Source: CAD feature listing. Evaluate the final solid. Frame: model axes, mm. Face numbers are marked on the shaded views. A direction names the side the tool comes from. Round coordinates to 2 decimals unless told otherwise and drop trailing zeros. Write each loop counter-clockwise with the first axis right and the second up, starting at its lowest first coordinate (ties: lowest second). Pieces come first, ordered by that corner, then holes. Notation, with made-up numbers: M -38,26 L -5,26 A20 ccw -5,30 Z; hole C 71.5,87.25 d9. An arc over 180 degrees is marked long. Put each result on its own line as item: value. Start each with the question number.
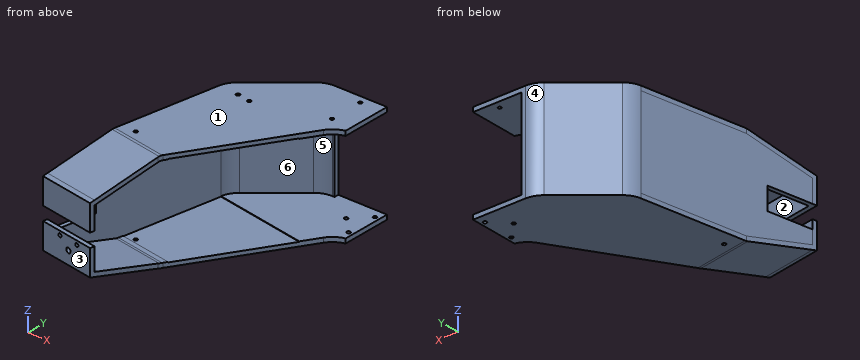
```python
from build123d import *

# Parameters (mm, degrees)
EXTRUDE_1_DEPTH      = 20
CUT_EXTRUDE_1_DEPTH  = 2
EXTRUDE_START        = 2
EXTRUDE_2_DEPTH      = 2
EXTRUDE_3_DEPTH      = 33
CUT_EXTRUDE_10_DEPTH = 22.5
EXTRUDE_4_DEPTH      = 25
SKETCH_19_W          = 6
SKETCH_19_H          = 22
CUT_EXTRUDE_11_DEPTH = 84.590810023
CUT_EXTRUDE_7_REACH  = 84.162
SKETCH_15_R          = 0.75
CUT_EXTRUDE_8_REACH  = 84.162
SKETCH_16_R          = 0.8
CUT_EXTRUDE_9_REACH  = 117.914
SKETCH_17_W          = 21.713584054
SKETCH_17_H          = 40
CUT_EXTRUDE_13_REACH = 84.162
SKETCH_23_R          = 0.8
SKETCH_24_R          = 0.8
CUT_EXTRUDE_14_DEPTH = 83.162435205
SKETCH_25_W          = 4
SKETCH_25_H          = 20
CUT_EXTRUDE_15_DEPTH = 82.996087258
CUT_EXTRUDE_16_REACH = 121.797
SKETCH_26_R          = 0.8
CUT_EXTRUDE_17_REACH = 121.797
SKETCH_27_R          = 1.1
FILLET_1_R           = 5
FILLET_2_R           = 5
FILLET_3_R           = 5
CUT_EXTRUDE_18_DEPTH = 20.2


with BuildPart() as part:
    # 草图1 → 凸台-拉伸1 (new, symmetric)
    with BuildSketch(Plane.XY):
        with BuildLine():
            Line((20.657346874, 53.638724152), (44.017644532, 53.638724152))
            Line((44.017644532, 53.638724152), (44.017644532, 51.638724152))
            Line((44.017644532, 51.638724152), (21.385287343, 51.638724152))
            ThreePointArc((21.385287343, 51.638724152), (17.96508591, 51.03565036), (14.957411246, 49.299168583))
            Line((14.957411246, 49.299168583), (-4.39648281, 33.059323219))
            ThreePointArc((-4.39648281, 33.059323219), (-6.628860751, 30.398878788), (-7.816684243, 27.135360565))
            Line((-7.816684243, 27.135360565), (-20.950105242, -47.347971173))
            Line((-20.950105242, -47.347971173), (-22.919720748, -47.000674818))
            Line((-22.919720748, -47.000674818), (-9.659894213, 28.199538337))
            ThreePointArc((-9.659894213, 28.199538337), (-8.472070721, 31.463056561), (-6.23969278, 34.123500992))
            Line((-6.23969278, 34.123500992), (14.229470778, 51.299168583))
            ThreePointArc((14.229470778, 51.299168583), (17.237145441, 53.03565036), (20.657346874, 53.638724152))
        make_face()
    extrude(amount=EXTRUDE_1_DEPTH, both=True)

    # 草图3 → 切除-拉伸1 (cut)
    with BuildSketch(Plane(origin=(-14.191017833, 2.502259328, 0), x_dir=(0, 0, 1), z_dir=(-0.9848077530122074, 0.17364817766693458, 0))):
        Polygon((13, -50.266596698), (20, -50.266596698), (20, -20.906299041), align=None)
    cut_extrude_1 = extrude(amount=-CUT_EXTRUDE_1_DEPTH, mode=Mode.SUBTRACT)

    # 镜向1: 切除-拉伸1 across plane
    add(cut_extrude_1.mirror(Plane.XY), mode=Mode.SUBTRACT)

    # 草图4 → 凸台-拉伸2 (add)
    with BuildSketch(Plane.XY.offset(20).offset(EXTRUDE_START)):
        with BuildLine():
            Line((44.017644532, 53.638724152), (44.017644532, 31.638724152))
            ThreePointArc((44.017644532, 31.638724152), (40.473292143, 30.034681338), (37.809285693, 27.199464091))
            Line((37.809285693, 27.199464091), (6.798835262, -22.427630496))
            Line((6.798835262, -22.427630496), (-17.821358564, -18.086426054))
            Line((-17.821358564, -18.086426054), (-9.659894213, 28.199538337))
            ThreePointArc((-9.659894213, 28.199538337), (-8.472070721, 31.463056561), (-6.23969278, 34.123500992))
            Line((-6.23969278, 34.123500992), (14.229470778, 51.299168583))
            ThreePointArc((14.229470778, 51.299168583), (17.237145441, 53.03565036), (20.657346874, 53.638724152))
            Line((20.657346874, 53.638724152), (44.017644532, 53.638724152))
        make_face()
    extrude_2 = extrude(amount=-EXTRUDE_2_DEPTH)

    # 草图5 → 凸台-拉伸3 (add)
    with BuildSketch(Plane(origin=(-14.191017833, 2.502259328, 0), x_dir=(0, 0, 1), z_dir=(-0.9848077530122074, 0.17364817766693458, 0))):
        Polygon((22, -20.906299041), (15, -50.266596698), (13, -50.266596698), (20, -20.906299041), align=None)
    extrude_3 = extrude(amount=-EXTRUDE_3_DEPTH)

    # 镜向3: 凸台-拉伸2, 凸台-拉伸3 across plane
    add(extrude_2.mirror(Plane.XY))
    add(extrude_3.mirror(Plane.XY))

    # 草图18 → 切除-拉伸10 (cut, symmetric)
    with BuildSketch(Plane.XY):
        Polygon((6.798835262, -22.427630496), (1.700473078, -51.34187926), (9.578935102, -52.731064681), (14.677297286, -23.816815917), align=None)
    extrude(amount=CUT_EXTRUDE_10_DEPTH, both=True, mode=Mode.SUBTRACT)

    # 草图10 → 凸台-拉伸4 (add)
    with BuildSketch(Plane(origin=(-14.191017833, 2.502259328, 0), x_dir=(0, 0, 1), z_dir=(-0.9848077530122074, 0.17364817766693458, 0))):
        Polygon((-15, -50.266596698), (15, -50.266596698), (14.523165597, -52.266596698), (-14.523165597, -52.266596698), align=None)
    extrude(amount=-EXTRUDE_4_DEPTH)

    # 草图19 → 切除-拉伸11 (cut, through all)
    with BuildSketch(Plane(origin=(-14.191017833, 2.502259328, 0), x_dir=(0, 0, 1), z_dir=(-0.9848077530122074, 0.17364817766693458, 0))):
        with Locations((0, -41.266596698)):
            Rectangle(SKETCH_19_W, SKETCH_19_H)
    extrude(amount=-CUT_EXTRUDE_11_DEPTH, mode=Mode.SUBTRACT)

    # 草图15 → 切除-拉伸7 (cut, up to next)
    with BuildSketch(Plane.XY.offset(22), mode=Mode.PRIVATE) as cut_extrude_7_sk1:
        with Locations((35.017644532, 50.138724152)):
            Circle(SKETCH_15_R)
    cut_extrude_7_tool1 = extrude(cut_extrude_7_sk1.sketch, amount=-CUT_EXTRUDE_7_REACH, mode=Mode.PRIVATE) & part.part
    # 草图15 → 切除-拉伸7 (cut, up to next)
    with BuildSketch(Plane.XY.offset(22), mode=Mode.PRIVATE) as cut_extrude_7_sk2:
        with Locations((35.017644532, 35.138724152)):
            Circle(SKETCH_15_R)
    cut_extrude_7_tool2 = extrude(cut_extrude_7_sk2.sketch, amount=-CUT_EXTRUDE_7_REACH, mode=Mode.PRIVATE) & part.part
    add(cut_extrude_7_tool1.solids().sort_by_distance((35.017645, 50.138724, 22))[0], mode=Mode.SUBTRACT)
    add(cut_extrude_7_tool2.solids().sort_by_distance((35.017645, 35.138724, 22))[0], mode=Mode.SUBTRACT)

    # 草图16 → 切除-拉伸8 (cut, up to next)
    with BuildSketch(Plane(origin=(0, 0, -22), x_dir=(-1, 0, 0), z_dir=(0, 0, -1)), mode=Mode.PRIVATE) as cut_extrude_8_sk1:
        with Locations((-42.017644532, 49.638724152)):
            Circle(SKETCH_16_R)
    cut_extrude_8_tool1 = extrude(cut_extrude_8_sk1.sketch, amount=-CUT_EXTRUDE_8_REACH, mode=Mode.PRIVATE) & part.part
    # 草图16 → 切除-拉伸8 (cut, up to next)
    with BuildSketch(Plane(origin=(0, 0, -22), x_dir=(-1, 0, 0), z_dir=(0, 0, -1)), mode=Mode.PRIVATE) as cut_extrude_8_sk2:
        with Locations((-42.017644532, 35.638724152)):
            Circle(SKETCH_16_R)
    cut_extrude_8_tool2 = extrude(cut_extrude_8_sk2.sketch, amount=-CUT_EXTRUDE_8_REACH, mode=Mode.PRIVATE) & part.part
    # 草图16 → 切除-拉伸8 (cut, up to next)
    with BuildSketch(Plane(origin=(0, 0, -22), x_dir=(-1, 0, 0), z_dir=(0, 0, -1)), mode=Mode.PRIVATE) as cut_extrude_8_sk3:
        with Locations((-35.017644532, 42.638724152)):
            Circle(SKETCH_16_R)
    cut_extrude_8_tool3 = extrude(cut_extrude_8_sk3.sketch, amount=-CUT_EXTRUDE_8_REACH, mode=Mode.PRIVATE) & part.part
    add(cut_extrude_8_tool1.solids().sort_by_distance((42.017645, 49.638724, -22))[0], mode=Mode.SUBTRACT)
    add(cut_extrude_8_tool2.solids().sort_by_distance((42.017645, 35.638724, -22))[0], mode=Mode.SUBTRACT)
    add(cut_extrude_8_tool3.solids().sort_by_distance((35.017645, 42.638724, -22))[0], mode=Mode.SUBTRACT)

    # 草图17 → 切除-拉伸9 (cut, up to next)
    with BuildSketch(Plane.XZ.offset(-51.638724152), mode=Mode.PRIVATE) as cut_extrude_9_sk1:
        with Locations((33.160852505, 0)):
            Rectangle(SKETCH_17_W, SKETCH_17_H)
    cut_extrude_9_tool1 = extrude(cut_extrude_9_sk1.sketch, amount=-CUT_EXTRUDE_9_REACH, mode=Mode.PRIVATE) & part.part
    add(cut_extrude_9_tool1.solids().sort_by_distance((33.160853, 51.638724, 0))[0], mode=Mode.SUBTRACT)

    # 草图23 → 切除-拉伸13 (cut, up to next)
    with BuildSketch(Plane.XY.offset(22), mode=Mode.PRIVATE) as cut_extrude_13_sk1:
        with Locations((-0.619145661, 27.643236889)):
            Circle(SKETCH_23_R)
    cut_extrude_13_tool1 = extrude(cut_extrude_13_sk1.sketch, amount=-CUT_EXTRUDE_13_REACH, mode=Mode.PRIVATE) & part.part
    # 草图23 → 切除-拉伸13 (cut, up to next)
    with BuildSketch(Plane.XY.offset(22), mode=Mode.PRIVATE) as cut_extrude_13_sk2:
        with Locations((5.289700857, 26.601347823)):
            Circle(SKETCH_23_R)
    cut_extrude_13_tool2 = extrude(cut_extrude_13_sk2.sketch, amount=-CUT_EXTRUDE_13_REACH, mode=Mode.PRIVATE) & part.part
    add(cut_extrude_13_tool1.solids().sort_by_distance((-0.619146, 27.643237, 22))[0], mode=Mode.SUBTRACT)
    add(cut_extrude_13_tool2.solids().sort_by_distance((5.289701, 26.601348, 22))[0], mode=Mode.SUBTRACT)

    # 草图24 → 切除-拉伸14 (cut, through all)
    with BuildSketch(Plane.XY.offset(22)):
        with Locations((-10.595826096, -14.770754093)):
            Circle(SKETCH_24_R)
    extrude(amount=-CUT_EXTRUDE_14_DEPTH, mode=Mode.SUBTRACT)

    # 草图25 → 切除-拉伸15 (cut, through all)
    with BuildSketch(Plane(origin=(-12.221402327, 2.154962972, 0), x_dir=(0, 0, -1), z_dir=(0.9848077530122075, -0.1736481776669347, 0))):
        with Locations((5, -40.266596698)):
            Rectangle(SKETCH_25_W, SKETCH_25_H)
    extrude(amount=-CUT_EXTRUDE_15_DEPTH, mode=Mode.SUBTRACT)

    # 草图26 → 切除-拉伸16 (cut, up to next)
    with BuildSketch(Plane(origin=(-9.075999269, -51.472549652, 0), x_dir=(0.9848077530122074, -0.17364817766693458, 0), z_dir=(-0.17364817766693458, -0.9848077530122074, 0)), mode=Mode.PRIVATE) as cut_extrude_16_sk1:
        with Locations((3.590062842, -4.75)):
            Circle(SKETCH_26_R)
    cut_extrude_16_tool1 = extrude(cut_extrude_16_sk1.sketch, amount=-CUT_EXTRUDE_16_REACH, mode=Mode.PRIVATE) & part.part
    # 草图26 → 切除-拉伸16 (cut, up to next)
    with BuildSketch(Plane(origin=(-9.075999269, -51.472549652, 0), x_dir=(0.9848077530122074, -0.17364817766693458, 0), z_dir=(-0.17364817766693458, -0.9848077530122074, 0)), mode=Mode.PRIVATE) as cut_extrude_16_sk2:
        with Locations((-5.409937158, -4.75)):
            Circle(SKETCH_26_R)
    cut_extrude_16_tool2 = extrude(cut_extrude_16_sk2.sketch, amount=-CUT_EXTRUDE_16_REACH, mode=Mode.PRIVATE) & part.part
    add(cut_extrude_16_tool1.solids().sort_by_distance((-5.540478, -52.095958, -4.75))[0], mode=Mode.SUBTRACT)
    add(cut_extrude_16_tool2.solids().sort_by_distance((-14.403747, -50.533124, -4.75))[0], mode=Mode.SUBTRACT)

    # 草图27 → 切除-拉伸17 (cut, up to next)
    with BuildSketch(Plane(origin=(-9.075999269, -51.472549652, 0), x_dir=(0.9848077530122074, -0.17364817766693458, 0), z_dir=(-0.17364817766693458, -0.9848077530122074, 0)), mode=Mode.PRIVATE) as cut_extrude_17_sk1:
        with Locations((-0.909937158, -8.75)):
            Circle(SKETCH_27_R)
    cut_extrude_17_tool1 = extrude(cut_extrude_17_sk1.sketch, amount=-CUT_EXTRUDE_17_REACH, mode=Mode.PRIVATE) & part.part
    add(cut_extrude_17_tool1.solids().sort_by_distance((-9.972112, -51.314541, -8.75))[0], mode=Mode.SUBTRACT)

    # 圆角1
    fillet_1_edges = [part.edges().sort_by_distance(p)[0] for p in [
        (-5.511261651, -20.257028275, -22),
        (-5.511261651, -20.257028275, 22),
    ]]
    fillet(fillet_1_edges, radius=FILLET_1_R)

    # 圆角2
    fillet_2_edges = [part.edges().sort_by_distance(p)[0] for p in [
        (-4.526453898, -20.430676453, -20),
        (-4.526453898, -20.430676453, 20),
    ]]
    fillet(fillet_2_edges, radius=FILLET_2_R)

    # 圆角3
    fillet_3_edges = [part.edges().sort_by_distance(p)[0] for p in [
        (6.798835262, -22.427630496, 20.965328277),
        (6.798835262, -22.427630496, -20.965328277),
    ]]
    fillet(fillet_3_edges, radius=FILLET_3_R)

    # 草图28 → 切除-拉伸18 (cut, symmetric)
    with BuildSketch(Plane.XY):
        Polygon((-15.402375378, -15.885231658), (-7.816684243, 27.135360565), (37.188945048, 19.199653837), (27.398461996, -23.432174084), align=None)
    extrude(amount=CUT_EXTRUDE_18_DEPTH, both=True, mode=Mode.SUBTRACT)


solid = part.part
```
(1) Contact query for flat-ended pins moving along their axis: P1, Ø2, axis at x = -8, z = 14.5, coming from the -Y side; P2, Ø1.3, axis at x = 42.02, y = 35.64, coming from the -Z side; P3, Ø1.5, axis at x = 18.5, z = -14, coming from the -Y side. Output: stop coordinate, or through.
(2) Section query A-A (y = -44). Return loops of the section in (x, z), and give its area (3 significant figures).
(3) Section query B-B (z = 1.5). Return loops of the section in (x, y).
(4) Ray query, line 1 along Z through (x, y) = (36.5, 43.5); line 2 along Z through (x, y) = (-10.5, 3.5); line 3 along X through (y, z) = (-16, 1.5). Return the intervals inside material, ascending.
(5) Section query D-D (y = 39.5). Return loops of the section in (x, z).
(6) Pull-direction query (Z, two-part tool) for the marked faces 1, 2 and 3; classes: +Z half, -Z half, draft (parallel to the pull), parting line (faces both ways), or undercut.
(7) Section query C-C (x = 32). Return loops of the section in (y, z).
(8) Access query for the marked faces 4, 5 and 6. Directions: +Z, -Z, +X, -X, +Y, -Y. A direction counts if a zero-diameter tool reaches every point of the face in a straight line with its end or side. Return the directions, or none.
Entries:
1. P1: y = -51.84
1. P2: z = 20
1. P3: y = 50.95
2. outline: M -22.39,-15.73 L 3,-16.78 L 3,-14.78 L -20.36,-13.81 L -20.36,-7 L -22.39,-7 Z; M -22.39,3 L -20.36,3 L -20.36,13.81 L 3,14.78 L 3,16.78 L -22.39,15.73 Z
2. area: 137 mm2
3. outline: M -19.45,-27.3 L -17.48,-27.65 L -7.82,27.14 A10 cw -4.4,33.06 L 14.96,49.3 A10 cw 21.39,51.64 L 22.3,51.64 L 22.3,53.64 L 20.66,53.64 A10 ccw 14.23,51.3 L -6.24,34.12 A10 ccw -9.66,28.2 Z
4. line 1: -22 to -20, 20 to 22
4. line 2: -22 to -20.2, 20.2 to 22
4. line 3: -17.45 to -15.42
5. outline: M 0.17,-22 L 44.02,-22 L 44.02,-20 L 3.28,-20 L 3.28,20 L 44.02,20 L 44.02,22 L 0.17,22 Z
6. face 1: +Z half
6. face 2: undercut
6. face 3: draft
7. outline: M 17.9,-22 L 53.64,-22 L 53.64,-20 L 20.11,-20 L 20.11,-20.2 L 17.9,-20.2 Z; M 17.9,20.2 L 20.11,20.2 L 20.11,20 L 53.64,20 L 53.64,22 L 17.9,22 Z
8. face 4: +Z, -Z, -X, +Y
8. face 5: +X, -Y
8. face 6: +X
